from build123d import *

# Parameters (mm, degrees)
F0_W     = 100
F0_H     = 80
F1_DEPTH = 40
F3_DEPTH = 6
F4_R     = 7
F5_W     = 95.5
F5_H     = 75.5
F5_W_2   = 92
F5_H_2   = 72
F6_DEPTH = 1.25
F7_R     = 2
F8_DEPTH = 25


with BuildPart() as f1:
    # F0 (on Top) → F1 (new body)
    with BuildSketch(Plane.XY):
        with Locations((50, 40)):
            Rectangle(F0_W, F0_H)
        Polygon((85, 4), (15, 4), (15, 15), (4, 15), (4, 65), (15, 65), (15, 76), (85, 76), (85, 65), (96, 65), (96, 15), (85, 15), align=None, mode=Mode.SUBTRACT)
    extrude(amount=F1_DEPTH)

    # F2 (on face) → F3 (join)
    with BuildSketch(Plane(origin=(0, 0, 0), x_dir=(1, 0, 0), z_dir=(0, 0, -1))):
        with BuildLine():
            Line((120, 0), (-20, 0))
            Line((-20, 0), (-20, -11.875))
            Line((-20, -11.875), (-6, -11.875))
            ThreePointArc((-6, -11.875), (-2.875, -15), (-6, -18.125))
            Line((-6, -18.125), (-20, -18.125))
            Line((-20, -18.125), (-20, -61.875))
            Line((-20, -61.875), (-6, -61.875))
            ThreePointArc((-6, -61.875), (-2.875, -65), (-6, -68.125))
            Line((-6, -68.125), (-20, -68.125))
            Line((-20, -68.125), (-20, -80))
            Line((-20, -80), (120, -80))
            Line((120, -80), (120, -68.125))
            Line((120, -68.125), (106, -68.125))
            ThreePointArc((106, -68.125), (102.875, -65), (106, -61.875))
            Line((106, -61.875), (120, -61.875))
            Line((120, -61.875), (120, -18.125))
            Line((120, -18.125), (106, -18.125))
            ThreePointArc((106, -18.125), (102.875, -15), (106, -11.875))
            Line((106, -11.875), (120, -11.875))
            Line((120, -11.875), (120, 0))
        make_face()
    extrude(amount=F3_DEPTH)

    # F4
    f4_edges = [f1.edges().sort_by_distance(p)[0] for p in [
        (15, 65, 20),
        (15, 15, 20),
        (85, 65, 20),
        (85, 15, 20),
    ]]
    fillet(f4_edges, radius=F4_R)

    # F5 (on face) → F6 (join)
    with BuildSketch(Plane.XY.offset(40)):
        with Locations((50, 40)):
            Rectangle(F5_W, F5_H)
        with Locations((50, 40)):
            Rectangle(F5_W_2, F5_H_2, mode=Mode.SUBTRACT)
    extrude(amount=F6_DEPTH)

    # F7 (on face) → F8 (cut)
    with BuildSketch(Plane.XY.offset(40)):
        with Locations((9, 9)):
            Circle(F7_R)
        with Locations((9, 70.342632)):
            Circle(F7_R)
        with Locations((91, 71)):
            Circle(F7_R)
        with Locations((91, 9)):
            Circle(F7_R)
    extrude(amount=-F8_DEPTH, mode=Mode.SUBTRACT)


solid = f1.part
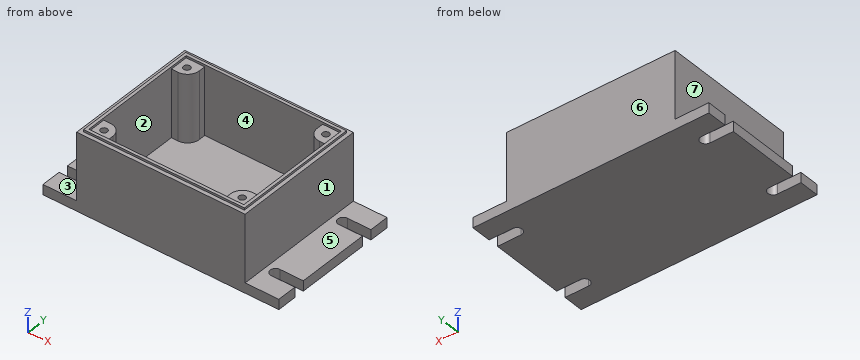
Build history of the part. All positions in model axes, mm. Face numbers are marked on the shaded views. A direction names the side the tool comes from. Coordinates: 2 decimals unless noted, no trailing zeros. Write each loop counter-clockwise with the first axis right and the second up, starting at its lowest first coordinate (ties: lowest second). Pieces come first, ordered by that corner, then holes.
(1) Cut at D-D on x = 30. List the corners of the cut face in (y, z), and give its area (3 significant figures).
(2) 3-axis set-ups, long thin cutter, end or side, ignore diameter. For the marked faces 4, 5, 6 and 7: which of +Z, -Z, +X, -X, +Y, -Y reach the whole face in a straight line?
(3) Drill centre lines: line 1 (X direction, y = 52, z = 31); line 2 (Y direction, x = 9, z = 28.25); line 3 (Y direction, x = 91, z = 22). Where is each one in solid material? Low to high.
(4) Cut at C-C on z = 35.5. List the corners of the cut face in (x, y), and give its area (3 significant figures).
(5) Pin check, flat tips, straight feed: pin 1 Ø4.5 at (y, z) = (73.5, 13) entering from -X; pin 2 Ø3 at (x, y) = (78.5, 54.5) entering from +Z; pin 3 Ø2 at (y, z) = (6, 10) entering from +X. Stop position of each tip, or through.
(6) Cut at B-B on y = 51. List the corners of the cut face in (x, z).
(7) Cut at A-A on x = 110. List the corners of the cut face in (y, z) (3 decimals), and give its area (3 significant figures).
(8) Mould opens along X. For the marked faces 1, 2 and 3 say: pulls with the +X half, pulls with the -X half, needs draft (parallel to the pull), parting line crosses it, or undercut.
Working result:
1. outline: (0, -6) - (80, -6) - (80, 40) - (77.75, 40) - (77.75, 41.25) - (76, 41.25) - (76, 0) - (4, 0) - (4, 41.25) - (2.25, 41.25) - (2.25, 40) - (0, 40) - close
1. area: 804 mm2
2. face 4: +Z
2. face 5: +Z, +X, +Y, -Y
2. face 6: +Z, -Z, +X, -X, +Y
2. face 7: +Z, -X, +Y, -Y
3. line 1: x = 0 to 4, 96 to 100
3. line 2: y = 0 to 7, 11 to 14.93, 65.07 to 68.34, 72.34 to 80
3. line 3: y = 0 to 7, 11 to 14.93, 65.07 to 69, 73 to 80
4. outline: (0, 0) - (100, 0) - (100, 80) - (0, 80) - close; hole (4, 15) - (8, 15) arc R7 cw to (15, 8) - (15, 4) - (85, 4) - (85, 8) arc R7 cw to (92, 15) - (96, 15) - (96, 65) - (92, 65) arc R7 cw to (85, 72) - (85, 76) - (15, 76) - (15, 72) arc R7 cw to (8, 65) - (4, 65) - close; hole circle Ø4 at (9, 9); hole circle Ø4 at (9, 70.34); hole circle Ø4 at (91, 9); hole circle Ø4 at (91, 71)
4. area: 1,770 mm2
5. pin 1: stops at x = 0
5. pin 2: stops at z = 0
5. pin 3: stops at x = 100
6. outline: (-20, -6) - (120, -6) - (120, 0) - (100, 0) - (100, 40) - (97.75, 40) - (97.75, 41.25) - (96, 41.25) - (96, 0) - (4, 0) - (4, 41.25) - (2.25, 41.25) - (2.25, 40) - (0, 40) - (0, 0) - (-20, 0) - close
7. outline: (0, -6) - (11.875, -6) - (11.875, 0) - (0, 0) - close; (18.125, -6) - (61.875, -6) - (61.875, 0) - (18.125, 0) - close; (68.125, -6) - (80, -6) - (80, 0) - (68.125, 0) - close
7. area: 405 mm2
8. face 1: pulls with the +X half
8. face 2: undercut
8. face 3: needs draft
